Input: part model. Units: mm. Frame: model coordinates. Coordinates: 2 decimals unless noted, no trailing zeros. Order: outer loops, then holes, each group sorted by start corner. A loop starts at its lowest first (then second) coordinate and runs counter-clockwise, first axis right, second up.
from build123d import *

# Parameters (mm, degrees)
SKETCH_2_R      = 2.1
SKETCH_2_R_2    = 3.1
EXTRUDE_1_DEPTH = 4
FILLET_1_R      = 5


with BuildPart() as part:
    # 草图2 → 凸台-拉伸1 (new body)
    with BuildSketch(Plane.XY):
        with BuildLine():
            Line((-14.5, 14.75), (-37.104267152, -37.841226517))
            ThreePointArc((-37.104267152, -37.841226517), (-35.091941928, -45.180309644), (-27.489316181, -44.846130471))
            Line((-27.489316181, -44.846130471), (7, -14.75))
            Line((7, -14.75), (7, 14.75))
            Line((7, 14.75), (-14.5, 14.75))
        make_face()
        with Locations((-4, 9)):
            Circle(SKETCH_2_R, mode=Mode.SUBTRACT)
        with Locations((-4, -9)):
            Circle(SKETCH_2_R, mode=Mode.SUBTRACT)
        with Locations((-31.5, -40.25)):
            Circle(SKETCH_2_R_2, mode=Mode.SUBTRACT)
    extrude(amount=EXTRUDE_1_DEPTH)

    # 圆角1
    fillet_1_edges = [part.edges().sort_by_distance(p)[0] for p in [
        (-14.5, 14.75, 2),
        (7, 14.75, 2),
        (7, -14.75, 2),
    ]]
    fillet(fillet_1_edges, radius=FILLET_1_R)


solid = part.part
Item 1: Ray query, probe 1 along Y at (x, z) = (-3, 3.3); probe 2 along Y at (x, z) = (-4, 1.15); probe 3 along Y at (x, z) = (-33, 2.75). Return the intervals inside material, ascending.
Response values:
probe 1: y = -23.48 to -10.85, -7.15 to 7.15, 10.85 to 14.75
probe 2: y = -24.35 to -11.1, -6.9 to 6.9, 11.1 to 14.75
probe 3: y = -46.16 to -42.96, -37.54 to -28.29
Item 2: Cut plane B-B on y = -9. Return loops of the section in (x, z), then the cut area to 3 significant figures.
Response values:
outline: (-24.71, 0) - (-6.1, 0) - (-6.1, 4) - (-24.71, 4) - close; (-1.9, 0) - (7, 0) - (7, 4) - (-1.9, 4) - close
area: 110 mm2
Item 3: Cut plane A-A on z = 1.8. Return loops of the section in (x, y).
Response values:
outline: (-37.1, -37.84) arc R6.1 ccw to (-27.49, -44.85) - (5.29, -16.24) arc R5 ccw to (7, -12.48) - (7, 9.75) arc R5 ccw to (2, 14.75) - (-11.21, 14.75) arc R5 ccw to (-15.8, 11.72) - close; hole circle Ø6.2 at (-31.5, -40.25); hole circle Ø4.2 at (-4, -9); hole circle Ø4.2 at (-4, 9)
Item 4: Cut plane D-D on x = -31.5. Return loops of the section in (y, z), then the cut area to 3 significant figures.
Response values:
outline: (-46.35, 0) - (-43.35, 0) - (-43.35, 4) - (-46.35, 4) - close; (-37.15, 0) - (-24.8, 0) - (-24.8, 4) - (-37.15, 4) - close
area: 61.4 mm2
Item 5: Draft query along X for faces 1 (the face through (-11.33, -30.745, 1.972)), 2 (the face through (-4.273, -6.918, 1.972)), 3 (the face through (-35.2, -45.1, 2)). Return one class per face: pulls with the +X half, pulls with the -X half, needs draft (parallel to the pull), parting line crosses it, or undercut.
Response values:
face 1: pulls with the +X half
face 2: undercut
face 3: parting line crosses it
Item 6: Cut plane C-C on x = -4. Return loops of the section in (y, z).
Response values:
outline: (-24.35, 0) - (-11.1, 0) - (-11.1, 4) - (-24.35, 4) - close; (-6.9, 0) - (6.9, 0) - (6.9, 4) - (-6.9, 4) - close; (11.1, 0) - (14.75, 0) - (14.75, 4) - (11.1, 4) - close
